Input: part model. Units: mm. Frame: model coordinates. Coordinates: 2 decimals unless noted, no trailing zeros. Loops run counter-clockwise (first coordinate to the right, second up) from the corner with the lowest first, then second, coordinate; pieces in that order, holes last. Notation, with made-up numbers: M -21,-8 L -17,-8 A17 ccw -17,18 Z; hole C 32.25,9.25 d10. An arc over 180 degrees is marked long. Use a Markdown table: item, result. Add a question column.
1. Line query: L1, parallel to X at y = -2, z = 0; L2, parallel to Y at x = 0.9, z = -0.35; L3, parallel to X at y = 1.25, z = -0.1. Output: solid intervals per line, ascending. Write a range as [from, to].
2. Section B-B on x = 0. Output: boundary loops of the cut face in (y, z).
3. Section C-C on y = 0.75. Output: boundary loops of the cut face in (x, z), then the cut area to 3 significant figures.
4. Section D-D on y = -0.75. Output: boundary loops of the cut face in (x, z).
5. Section A-A on z = 0. Output: boundary loops of the cut face in (x, y), then the cut area to 3 significant figures.
6. Pin query (flat end, axial travel): pin 1 (1 mm diameter, centred on y = -2, z = 0.5, fed in from +X). Return the tip coordinate at first contact, or that it passes through.
```python
from build123d import *

# Parameters (mm, degrees)
SKETCH1_R           = 1.55
BOSS_EXTRUDE1_DEPTH = 5.4
SKETCH2_R           = 0.15783532
SKETCH2_R_2         = 0.131217629
BOSS_EXTRUDE2_DEPTH = 3.81


with BuildPart() as part:
    # Sketch1 → Boss-Extrude1 (new body)
    # profile 1 of 2: a face of its own
    with BuildSketch(Plane(origin=(0, 0, 0), x_dir=(1, 0, 0), z_dir=(0, 1, 0))):
        with BuildLine():
            Line((-1.010787693, -1.608822004), (1.010787693, -1.608822004))
            ThreePointArc((1.010787693, -1.608822004), (0, 1.9), (-1.010787693, -1.608822004))
        make_face()
        Circle(SKETCH1_R, mode=Mode.SUBTRACT)
    # profile 2 of 2: a face of its own
    with BuildSketch(Plane(origin=(0, 0, 0), x_dir=(1, 0, 0), z_dir=(0, 1, 0))):
        Circle(SKETCH1_R)
    extrude(amount=BOSS_EXTRUDE1_DEPTH)

    # Sketch2 → Boss-Extrude2 (add)
    with BuildSketch(Plane.XZ):
        with Locations(Location((0.904579412, 0, 0), (0, 0, 90))):
            Circle(SKETCH2_R)
        with Locations(Location((-0.93688582, 0, 0), (0, 0, 90))):
            Circle(SKETCH2_R_2)
    extrude(amount=BOSS_EXTRUDE2_DEPTH)


solid = part.part
```
Answers below:
| question | item | result |
|---|---|---|
| 1 | L1 | x = [-1.07, -0.81], [0.75, 1.06] |
| 1 | L2 | y = [0, 5.4] |
| 1 | L3 | x = [-1.9, 1.9] |
| 2 | outline | M 0,-1.9 L 5.4,-1.9 L 5.4,1.61 L 0,1.61 Z |
| 3 | outline | M -1.01,1.61 A1.9 ccw long 1.01,1.61 Z |
| 3 | area | 10.9 mm² |
| 4 | outline | C -0.94,0 d0.26; C 0.9,0 d0.32 |
| 5 | outline | M -1.9,0 L -1.07,0 L -1.07,-3.81 L -0.81,-3.81 L -0.81,0 L 0.75,0 L 0.75,-3.81 L 1.06,-3.81 L 1.06,0 L 1.9,0 L 1.9,5.4 L -1.9,5.4 Z |
| 5 | area | 22.7 mm² |
| 6 | pin 1 | stops at x = 1.06 |
